Check sheet for the modelled part. Datum: model origin and axes. Units: mm. Face numbers are marked on the shaded views. A direction names the side the tool comes from. Give positions to 0.01 mm unless a question says otherwise; leave off trailing zeros. Write each loop counter-clockwise with the first axis right and the second up, starting at its lowest first coordinate (ties: lowest second). Pieces come first, ordered by that corner, then holes. Notation, with made-up numbers: M 71,57 L 76,57 A3 ccw 76,61 Z; hole C 62,1.5 d11. An arc over 180 degrees is marked long. Write item = value, one per line. Start each with the question number.
1) Cross-section at A-A, the plane x = -23. Record the cut outline in (y, z), plus the area to 3 significant figures.
2) Access from +Z, -Z, +X, -X, +Y, -Y to the whole of each face (thin tool, end or side, straight path). Record for the marked faces 1 and 2.
3) Cross-section at D-D, the plane y = 3. Record the cut outline in (x, z) (3 decimals).
4) Cross-section at B-B, the plane x = -58.5. Record the cut outline in (y, z).
5) Mould release check, pull along Z, two halves, no side actions. Record for the marked faces 3, 4 and 5: released by +Z, released by -Z, zero draft, split by the parting line, or undercut.
6) Cross-section at C-C, the plane z = 50. Record the cut outline in (x, y), plus the area to 3 significant figures.
7) Go/stop test with flat-tipped pins: pin 1 (1.1 mm diameter, centred on x = -53.5, z = 40.5, fed in from +Y); pin 2 (1 mm diameter, centred on x = -29, z = 11, fed in from +Y); pin 3 (12 mm diameter, centred on y = -5, z = 83.5, fed in from -X); pin 4 (12 mm diameter, centred on x = -23.5, z = 43.5, fed in from +Y). Record where each tip stops, or that it passes through.
8) Scan lines: line 1 along Y through (x, z) = (-52, 61.5); line 2 along Y through (x, z) = (-42.5, 8); line 3 along X through (y, z) = (-1.5, 17.5). Record each from-to range of solid material in increasing order. Write a range as [from, to].
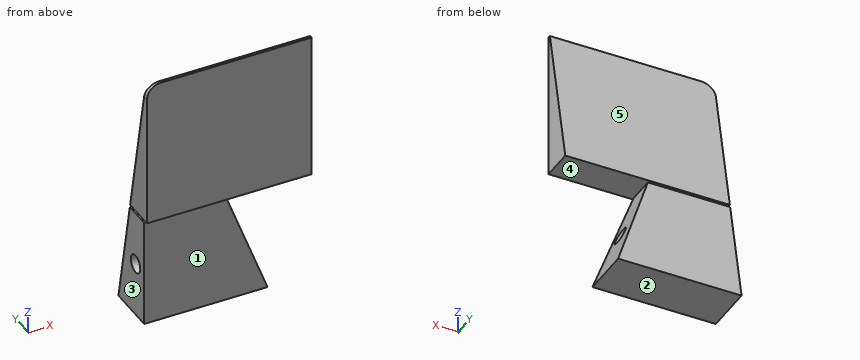
```python
from build123d import *

# Parameters (mm, degrees)
ESBO_O1_W                                      = 130
ESBO_O1_H                                      = 20
RESSALTO_EXTRUS_O1_DEPTH                       = 95
CORTE_EXTRUS_O2_REACH                          = 22
CORTE_EXTRUS_O4_DEPTH                          = 1
CORTE_EXTRUS_O4_DEPTH_BACK                     = 61
BROCA_DE_ROSQUEAR_DE_CANO_PARA_TARRAXA_D_D     = 6.579997
BROCA_DE_ROSQUEAR_DE_CANO_PARA_TARRAXA_D_DEPTH = 10
BROCA_DE_ROSQUEAR_DE_CANO_PARA_TARRAXA_D_TIP   = 1.976830535
BROCA_DE_ROSQUEAR_DE_CANO_PARA_TARRA_2_D       = 6.579997
BROCA_DE_ROSQUEAR_DE_CANO_PARA_TARRA_2_DEPTH   = 10
BROCA_DE_ROSQUEAR_DE_CANO_PARA_TARRA_2_TIP     = 1.976830535
FILETE2_R                                      = 5
CORTE_EXTRUS_O10_REACH                         = 62
RESSALTO_EXTRUS_O2_REACH                       = 57
ESBO_O41_W                                     = 28
ESBO_O41_H                                     = 8
ESBO_O42_W                                     = 45
ESBO_O42_H                                     = 2
CORTE_EXTRUS_O11_DEPTH                         = 41


with BuildPart() as part:
    # Esboço1 → Ressalto-extrusão1 (new body)
    with BuildSketch(Plane.XY):
        Rectangle(ESBO_O1_W, ESBO_O1_H)
    extrude(amount=RESSALTO_EXTRUS_O1_DEPTH)

    # Esboço2 → Corte-extrusão2 (cut, up to next)
    with BuildSketch(Plane(origin=(0, 10, 0), x_dir=(1, 0, 0), z_dir=(0, 1, 0)), mode=Mode.PRIVATE) as corte_extrus_o2_sk1:
        Polygon((65, 0), (-20, 0), (-35, -40), (-35, -41), (-5, -41), (-5, -95), (65, -95), align=None)
    corte_extrus_o2_tool1 = extrude(corte_extrus_o2_sk1.sketch, amount=-CORTE_EXTRUS_O2_REACH, mode=Mode.PRIVATE) & part.part
    add(corte_extrus_o2_tool1.solids().sort_by_distance((24.261214, 10, 44.470976))[0], mode=Mode.SUBTRACT)

    # Esboço13 → Corte-extrusão4 (cut, two sides)
    with BuildSketch(Plane.ZY.offset(65)) as corte_extrus_o4_sk:
        Polygon((-200.200134404, 50.040026881), (0, 10), (95, -9), (295.200134404, -49.040026881), (375.280188165, 351.360241926), (-120.120080642, 450.440295688), align=None)
    extrude(amount=CORTE_EXTRUS_O4_DEPTH, mode=Mode.SUBTRACT)
    extrude(corte_extrus_o4_sk.sketch, amount=-CORTE_EXTRUS_O4_DEPTH_BACK, mode=Mode.SUBTRACT)

    # Broca de rosquear de cano para tarraxa d
    with Locations(Plane.ZY.offset(65)):
        with Locations((20, -2)):
            Hole(BROCA_DE_ROSQUEAR_DE_CANO_PARA_TARRAXA_D_D / 2, depth=BROCA_DE_ROSQUEAR_DE_CANO_PARA_TARRAXA_D_DEPTH)
            with Locations((0, 0, -(BROCA_DE_ROSQUEAR_DE_CANO_PARA_TARRAXA_D_DEPTH + BROCA_DE_ROSQUEAR_DE_CANO_PARA_TARRAXA_D_TIP / 2))):  # 118° drill point
                Cone(0, BROCA_DE_ROSQUEAR_DE_CANO_PARA_TARRAXA_D_D / 2, BROCA_DE_ROSQUEAR_DE_CANO_PARA_TARRAXA_D_TIP, mode=Mode.SUBTRACT)

    # Broca de rosquear de cano para tarra 2
    with Locations(Plane(origin=(-17.534246575, 0, -6.575342466), x_dir=(0.351123442, 0, -0.936329178), z_dir=(0.936329178, 0, 0.351123442))):
        with Locations((-27.022468832, -2)):
            Hole(BROCA_DE_ROSQUEAR_DE_CANO_PARA_TARRA_2_D / 2, depth=BROCA_DE_ROSQUEAR_DE_CANO_PARA_TARRA_2_DEPTH)
            with Locations((0, 0, -(BROCA_DE_ROSQUEAR_DE_CANO_PARA_TARRA_2_DEPTH + BROCA_DE_ROSQUEAR_DE_CANO_PARA_TARRA_2_TIP / 2))):  # 118° drill point
                Cone(0, BROCA_DE_ROSQUEAR_DE_CANO_PARA_TARRA_2_D / 2, BROCA_DE_ROSQUEAR_DE_CANO_PARA_TARRA_2_TIP, mode=Mode.SUBTRACT)

    # Filete2
    filete2_edges = [part.edges().sort_by_distance(p)[0] for p in [
        (-65, -9.5, 95),
    ]]
    fillet(filete2_edges, radius=FILETE2_R)

    # Esboço40 → Corte-extrusão10 (cut, up to next)
    with BuildSketch(Plane.ZY.offset(65), mode=Mode.PRIVATE) as corte_extrus_o10_sk1:
        Polygon((41, 1.8), (41, -10), (40, -10), (40, 2), align=None)
    corte_extrus_o10_tool1 = extrude(corte_extrus_o10_sk1.sketch, amount=-CORTE_EXTRUS_O10_REACH, mode=Mode.PRIVATE) & part.part
    add(corte_extrus_o10_tool1.solids().sort_by_distance((-65, -4.04986, 40.498599))[0], mode=Mode.SUBTRACT)

    # Esboço41 → Ressalto-extrusão2 (add, up to next)
    with BuildSketch(Plane.XY.offset(40), mode=Mode.PRIVATE) as ressalto_extrus_o2_sk1:
        with Locations((-50, -3)):
            Rectangle(ESBO_O41_W, ESBO_O41_H)
    ressalto_extrus_o2_tool1 = extrude(ressalto_extrus_o2_sk1.sketch, amount=RESSALTO_EXTRUS_O2_REACH, mode=Mode.PRIVATE) - part.part
    add(ressalto_extrus_o2_tool1.solids().sort_by_distance((-50, -3, 40))[0])

    # Esboço42 → Corte-extrusão11 (cut)
    with BuildSketch(Plane(origin=(0, 0, 0), x_dir=(-1, 0, 0), z_dir=(0, 0, -1))):
        with Locations((42.5, -9)):
            Rectangle(ESBO_O42_W, ESBO_O42_H)
    extrude(amount=-CORTE_EXTRUS_O11_DEPTH, mode=Mode.SUBTRACT)


solid = part.part
```
Reply:
q1.outline = M -10,41 L 1.8,41 L -9,95 L -10,95 Z; M -8,0 L 10,0 L 8.4,8 L -8,8 Z
q1.area = 483 mm2
q2.face_1 = -Z, +X, -X, -Y
q2.face_2 = -Z, +X, -X, +Y, -Y
q3.outline = M -65,0 L -20,0 L -33.125,35 L -65,35 Z
q4.outline = M -10,41 L -7,41 L -7,40 L -8,40 L -8,0 L 10,0 L 2,40 L 1,40 L 1,41 L 1.8,41 L -9,95 L -10,95 Z; hole C -2,20 d6.58
q5.face_3 = zero draft
q5.face_4 = undercut
q5.face_5 = released by +Z
q6.outline = M -65,-10 L -5,-10 L -5,0 L -65,0 Z
q6.area = 600 mm2
q7.pin_1 = 2.01
q7.pin_2 = 7.9
q7.pin_3 = -65
q7.pin_4 = 1.8
q8.line_1 = [-10, -2.3]
q8.line_2 = [-8, 8.4]
q8.line_3 = [-54.56, -37.66]
